from build123d import *

# Parameters (mm, degrees)
F0_R     = 8.35
F1_DEPTH = 5


with BuildPart() as f1:
    # F0 (on Top) → F1 (new body)
    with BuildSketch(Plane.XY):
        with BuildLine():
            ThreePointArc((24.9799919936, -20), (30.1940370255, -10.5981190832), (32, 0))
            ThreePointArc((32, 0), (30.1940370255, 10.5981190832), (24.9799919936, 20))
            Line((24.9799919936, 20), (24.9799919936, 6.7116968793))
            Line((24.9799919936, 6.7116968793), (25.875, 6.7116968793))
            Line((25.875, 6.7116968793), (29.75, 0))
            Line((29.75, 0), (25.875, -6.7116968793))
            Line((25.875, -6.7116968793), (24.9799919936, -6.7116968793))
            Line((24.9799919936, -6.7116968793), (24.9799919936, -20))
        make_face()
        with BuildLine():
            Line((24.9799919936, 6.7116968793), (24.9799919936, 20))
            ThreePointArc((24.9799919936, 20), (16.5310257714, 11.0168846286), (7.0474671546, 18.9))
            Line((7.0474671546, 18.9), (6.8927707223, 18.9))
            ThreePointArc((6.8927707223, 18.9), (0, 13.0200080064), (-6.8927707223, 18.9))
            Line((-6.8927707223, 18.9), (-7.0474671546, 18.9))
            ThreePointArc((-7.0474671546, 18.9), (-16.5310257714, 11.0168846286), (-24.9799919936, 20))
            Line((-24.9799919936, 20), (-24.9799919936, 6.7116968793))
            Line((-24.9799919936, 6.7116968793), (-18.125, 6.7116968793))
            Line((-18.125, 6.7116968793), (-14.25, 0))
            Line((-14.25, 0), (-18.125, -6.7116968793))
            Line((-18.125, -6.7116968793), (-24.9799919936, -6.7116968793))
            Line((-24.9799919936, -6.7116968793), (-24.9799919936, -20))
            ThreePointArc((-24.9799919936, -20), (-12.7096008018, -11.75), (-0.43920961, -20))
            Line((-0.43920961, -20), (0.43920961, -20))
            ThreePointArc((0.43920961, -20), (12.7096008018, -11.75), (24.9799919936, -20))
            Line((24.9799919936, -20), (24.9799919936, -6.7116968793))
            Line((24.9799919936, -6.7116968793), (18.125, -6.7116968793))
            Line((18.125, -6.7116968793), (14.25, 0))
            Line((14.25, 0), (18.125, 6.7116968793))
            Line((18.125, 6.7116968793), (24.9799919936, 6.7116968793))
        make_face()
        Circle(F0_R, mode=Mode.SUBTRACT)
        with BuildLine():
            ThreePointArc((0, -21.2545297412), (0.2038636697, -20.6217539149), (0.43920961, -20))
            Line((0.43920961, -20), (-0.43920961, -20))
            ThreePointArc((-0.43920961, -20), (-0.2038636697, -20.6217539149), (0, -21.2545297412))
        make_face()
        with BuildLine():
            Line((-24.9799919936, 6.7116968793), (-24.9799919936, 20))
            ThreePointArc((-24.9799919936, 20), (-32, 0), (-24.9799919936, -20))
            Line((-24.9799919936, -20), (-24.9799919936, -6.7116968793))
            Line((-24.9799919936, -6.7116968793), (-25.875, -6.7116968793))
            Line((-25.875, -6.7116968793), (-29.75, 0))
            Line((-29.75, 0), (-25.875, 6.7116968793))
            Line((-25.875, 6.7116968793), (-24.9799919936, 6.7116968793))
        make_face()
    extrude(amount=F1_DEPTH)


solid = f1.part
Input: part model. Units: mm. Frame: model coordinates. A direction names the side the tool comes from. Coordinates: 2 decimals unless noted, no trailing zeros. Order: outer loops, then holes, each group sorted by start corner. A loop starts at its lowest first (then second) coordinate and runs counter-clockwise, first axis right, second up. Notation, with made-up numbers: M 59.5,-7.5 L 65.5,-7.5 A17 ccw 65.5,14.5 Z; hole C -10,83.25 d5. An arc over 180 degrees is marked long. Write item = value, one per line. Start each with the question number.
(1) First-contact query: P1, Ø1.5, axis at x = 23.5, z = 2.5, coming from the -Y side; P2, Ø2, axis at x = -10, z = 3.5, coming from the -Y side; P3, Ø1.5, axis at x = 22.5, z = 3, coming from the +Y side. Flat tips, straight axial feed; report the tip coordinate or a pass-through.
(2) Line query: line 1 along X through (y, z) = (2, 3.8); line 2 along X through (y, z) = (3.5, 1.2); line 3 along Y through (x, z) = (-29, 3.45). Output: solid intervals per line, ascending. Write a range as [from, to].
(3) Pull-direction query (Y, two-part tool) for faces 3 (the cylindrical face through (0.14, 13.02, 2.46)), 4 (the flat face through (27.84, -3.31, 2.46)), 5 (the flat face through (0, -10, 0)); classes: released by +Y, released by -Y, zero draft, split by the parting line, or undercut.
(4) Section A-A on z = 1.2. Output: boundary loops of the cut face in (x, y) (3 decimals).
(5) Section B-B on x = 4. Output: boundary loops of the cut face in (y, z), and give its area (3 significant figures).
(6) Section C-C on y = 14. Output: boundary loops of the cut face in (x, z), and give its area (3 significant figures).
(7) Reachability of faces 1 (the flat face through (22, 6.712, 2)), 2 (the cylindrical face through (16.72, 11.03, 2.46)) from +Z, -Z, +X, -X, +Y, -Y: full face, straight path, thin tool, end or side. Return the list, or none.
(8) Section D-D on x = -20. Output: boundary loops of the cut face in (y, z).
Result set:
q1.P1 = -18.49
q1.P2 = -12.28
q1.P3 = 14.69
q2.line_1 = [-31.94, -28.6], [-15.4, -8.11], [8.11, 15.4], [28.6, 31.94]
q2.line_2 = [-31.81, -27.73], [-16.27, -7.58], [7.58, 16.27], [27.73, 31.81]
q2.line_3 = [-13.53, -1.3], [1.3, 13.53]
q3.face_3 = released by +Y
q3.face_4 = undercut
q3.face_5 = zero draft
q4.outline = M -24.98,-20 A13.25 cw 0,-21.255 A13.25 cw 24.98,-20 A32 ccw 24.98,20 A9 cw 7.047,18.9 L 6.893,18.9 A6.98 cw -6.893,18.9 L -7.047,18.9 A9 cw -24.98,20 A32 ccw Z; hole M -29.75,0 L -25.875,-6.712 L -18.125,-6.712 L -14.25,0 L -18.125,6.712 L -25.875,6.712 Z; hole C 0,0 d16.7; hole M 14.25,0 L 18.125,-6.712 L 25.875,-6.712 L 29.75,0 L 25.875,6.712 L 18.125,6.712 Z
q5.outline = M -15.01,0 L -7.33,0 L -7.33,5 L -15.01,5 Z; M 7.33,0 L 14.28,0 L 14.28,5 L 7.33,5 Z
q5.area = 73.2 mm²
q6.outline = M -28.77,0 L -22.69,0 L -22.69,5 L -28.77,5 Z; M -9.27,0 L -3.57,0 L -3.57,5 L -9.27,5 Z; M 3.57,0 L 9.27,0 L 9.27,5 L 3.57,5 Z; M 22.69,0 L 28.77,0 L 28.77,5 L 22.69,5 Z
q6.area = 118 mm²
q7.face_1 = +Z, -Z
q7.face_2 = +Z, -Z, +Y
q8.outline = M -13.94,0 L -6.71,0 L -6.71,5 L -13.94,5 Z; M 6.71,0 L 11.95,0 L 11.95,5 L 6.71,5 Z
